Verification items for the finished model (mm, model axes). Coordinates: 2 decimals unless noted, no trailing zeros. Write each loop counter-clockwise with the first axis right and the second up, starting at its lowest first coordinate (ties: lowest second). Pieces come first, ordered by that corner, then holes. Notation, with made-up numbers: (-39.75, 11.25) - (-18.75, 11.25) arc R26 cw to (-18.75, 49.25) - close; hole circle Ø3 at (-18, -5). An arc over 180 degrees is marked (long way). Use one line per item in the form item = value. Start each with the question number.
(1) Sectioned sample at D-D (y = 0). Record the cut outline in (x, z), and give its area (3 significant figures).
(2) Sectioned sample at C-C (x = 0.9). Record the cut outline in (y, z).
(3) Gauge pin test, flat ends, axial feed: pin 1 Ø4 at (y, z) = (-25.87, 10.72) entering from -X; pin 2 Ø1 at (x, z) = (1, 5.5) entering from +Y. Record the tip position at first contact, or that the pin passes through.
(4) Material ranges on line 1 (Y direction, x = 0.45, z = 9.5); line 2 (Y direction, x = 2.8, z = 12); line 3 (Y direction, x = 1.8, z = 20.5), recorded low to high. Write a range as [from, to].
(5) Sectioned sample at B-B (z = 12). Record the cut outline in (x, y), and give its area (3 significant figures).
(6) Sectioned sample at A-A (z = 6.5). Record the cut outline in (x, y), and give its area (3 significant figures).
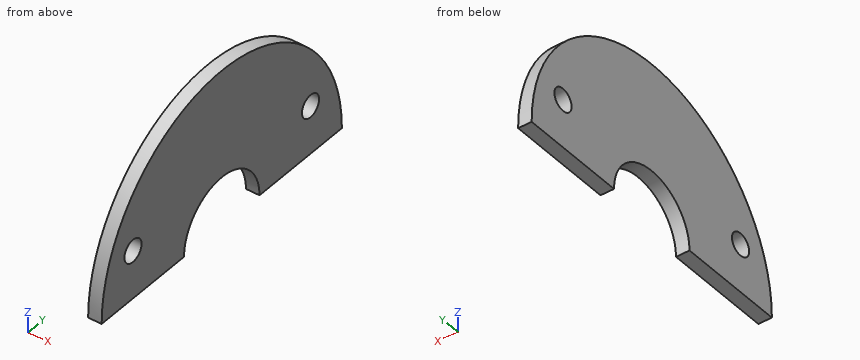
Autodesk Inventor part; units mm, degrees
ref_plane "YZ Plane" through (0, 0, 0) normal (1, 0, 0) x (0, 1, 0)
ref_plane "XZ Plane" through (0, 0, 0) normal (0, 1, 0) x (-1, 0, 0)
ref_plane "XY Plane" through (0, 0, 0) normal (0, 0, 1) x (1, 0, 0)
sketch "Sketch1" plane through (0, 0, 0) normal (1, 0, 0) x (0, 1, 0)
  circle A0 centre (0, 0) radius 35
  dimension "d0" = 70
extrude "Extrusion1" add sketch "Sketch1" along normal blind 3
sketch "Sketch2" plane through (3, 0, 0) normal (1, 0, 0) x (0, 0, -1)
  circle A0 centre (0, 0) radius 11
  circle A1 centre (0, 0) radius 35
  circle A2 centre (0, 0) radius 35
  line L0 (0, 35) -> (0, -35)
  point P0 (0, 11)
  point P1 (0, -11)
  dimension "d3" = 22
extrude "Extrusion2" cut sketch "Sketch2" against normal blind 3 contours A0 L0 | A0 L0 A1 | L0 A0 picked at (26.6156, -3.412)
sketch "Sketch3" plane through (3, 0, 0) normal (1, 0, 0) x (0, 0, -1)
  line L0 (0, 11) -> (0, 35)
  arc A0 (0, 35) -> (0, -35) centre (0, 0) ccw
  line L1 (0, -35) -> (0, -11)
  arc A1 (0, 11) -> (0, -11) centre (0, 0) ccw
  circle A2 centre (0, 0) radius 28 construction
  line L2 (0, 0) -> (-10.7151, 25.8686)
  line L3 (0, 0) -> (-10.7151, -25.8686)
  dimension "d6" = 56
  dimension "d7" = 22.5
  dimension "d8" = 22.5
hole "Hole1" at (3, 25.8686, 10.7151) at (3, -25.8686, 10.7151) direction (-1, 0, 0) diameter 5 end through all
properties part number "P004" material "Steel, Alloy"
Answers below:
q1.outline = (0, 11) - (3, 11) - (3, 35) - (0, 35) - close
q1.area = 72.0 mm2
q2.outline = (-35, 0) - (-11, 0) arc R11 cw to (11, 0) - (35, 0) arc R35 ccw to start; hole circle Ø5 at (-25.87, 10.72); hole circle Ø5 at (25.87, 10.72)
q3.pin_1 = through
q3.pin_2 = 34.64
q4.line_1 = [-33.69, -28.05], [-23.68, -5.55], [5.55, 23.68], [28.05, 33.69]
q4.line_2 = [-32.88, -28.01], [-23.72, 23.72], [28.01, 32.88]
q4.line_3 = [-28.37, 28.37]
q5.outline = (0, -32.88) - (3, -32.88) - (3, -28.01) - (0, -28.01) - close; (0, -23.72) - (3, -23.72) - (3, 23.72) - (0, 23.72) - close; (0, 28.01) - (3, 28.01) - (3, 32.88) - (0, 32.88) - close
q5.area = 172 mm2
q6.outline = (0, -34.39) - (3, -34.39) - (3, -8.87) - (0, -8.87) - close; (0, 8.87) - (3, 8.87) - (3, 34.39) - (0, 34.39) - close
q6.area = 153 mm2
